For this review, take the finished solid that the model builds, in its own axes (mm). Face numbers are marked on the shaded views. A direction names the side the tool comes from. Coordinates: 2 decimals unless noted, no trailing zeros. Write each loop counter-clockwise with the first axis right and the second up, starting at its lowest first coordinate (ties: lowest second). Pieces come first, ordered by that corner, then holes.
1) We need section C-C on z = -22. Write out the cut boundary in (x, y) (1 decimal).
2) For the marked faces 1 and 2, list the 3-axis set-ups (+Z, -Z, +X, -X, +Y, -Y) from which the entire face can be reached by the end or side of a thin tool; tool diameter is ignored.
3) Insertion check: P1, Ø2, axis at x = -2.5, y = 0, coming from the -Z side (3 decimals); P2, Ø1.5, axis at y = -2.5, z = -19, coming from the -X side (3 decimals). Each pin has a flat end and moves straight along its axis. Give the tip position at first contact, or say it passes through.
4) We need section B-B on x = 0.5. Write out the cut boundary in (y, z) (1 decimal), then the cut area to 3 significant figures.
5) We need section A-A on y = 0. Write out the cut boundary in (x, z) (1 decimal), then the cut area to 3 significant figures.
6) We need section D-D on y = -2.25. Write out the cut boundary in (x, z) (3 decimals), then the cut area to 3 significant figures.
7) To check wall thickness, follow line 1 along Z through (x, y) = (-1.75, -0.75) (3 decimals); line 2 along Y through (x, z) = (-0.5, -22); line 3 along Y through (x, z) = (-1, 1.5). State the ranges of each line that lie inside material, in increasing order.
from build123d import *

# Parameters (mm, degrees)
F0_R     = 3.175
F1_DEPTH = 3.175
F2_R     = 1.5875
F3_DEPTH = 34.925
F5_DEPTH = 2.38125


with BuildPart() as f1:
    # F0 (on Top) → F1 (new body)
    with BuildSketch(Plane.XY):
        Circle(F0_R)
    extrude(amount=F1_DEPTH)

    # F2 (on face) → F3 (join)
    with BuildSketch(Plane(origin=(0, 0, 0), x_dir=(1, 0, 0), z_dir=(0, 0, -1))):
        Circle(F2_R)
    extrude(amount=F3_DEPTH)

    # F4 (on face) → F5 (cut)
    with BuildSketch(Plane.XY.offset(3.175)):
        Polygon((1.50224, 1.050468), (-0.158612, 1.826212), (-1.660852, 0.775744), (-1.50224, -1.050468), (0.158612, -1.826212), (1.660852, -0.775744), align=None)
    extrude(amount=-F5_DEPTH, mode=Mode.SUBTRACT)


solid = f1.part
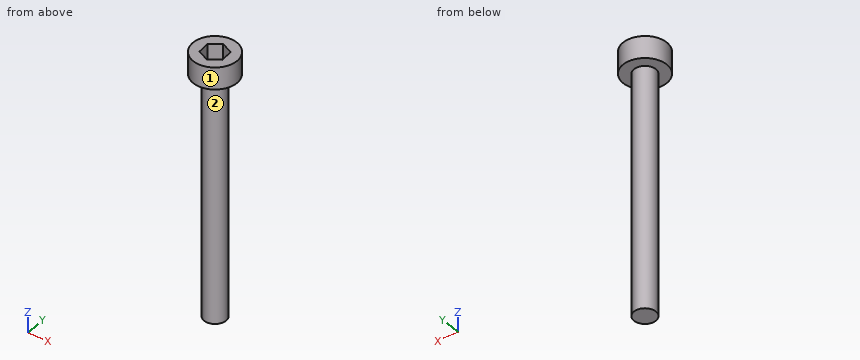
Result:
1. outline: circle Ø3.2 at (0, 0)
2. face 1: +Z, -Z
2. face 2: -Z
3. P1: stops at z = -34.925
3. P2: passes through
4. outline: (-3.1, 0) - (-1.5, 0) - (-1.5, -34.9) - (1.5, -34.9) - (1.5, 0) - (3.1, 0) - (3.1, 3.2) - (1.5, 3.2) - (1.5, 0.8) - (-1.6, 0.8) - (-1.6, 3.2) - (-3.1, 3.2) - close
4. area: 118 mm2
5. outline: (-3.2, 0) - (-1.6, 0) - (-1.6, -34.9) - (1.6, -34.9) - (1.6, 0) - (3.2, 0) - (3.2, 3.2) - (1.6, 3.2) - (1.6, 0.8) - (-1.6, 0.8) - (-1.6, 3.2) - (-3.2, 3.2) - close
5. area: 123 mm2
6. outline: (-2.24, 0) - (2.24, 0) - (2.24, 3.175) - (-2.24, 3.175) - close
6. area: 14.2 mm2
7. line 1: z = 0 to 3.175
7. line 2: y = -1.51 to 1.51
7. line 3: y = -3.01 to -1.29, 1.24 to 3.01
